Check sheet for the modelled part. Datum: model origin and axes. Units: mm. A direction names the side the tool comes from. Give positions to 0.01 mm unless a question says otherwise; leave off trailing zeros. Loops run counter-clockwise (first coordinate to the right, second up) from the corner with the lowest first, then second, coordinate; pieces in that order, holes last. Notation, with made-up numbers: (86, 78) -> (138, 78) arc R38 cw to (138, 116) -> close; hole circle Ø11 at (71, 64.25). An arc over 180 degrees is marked (long way). Answer as CSV lines item,"result". Start each with the question number.
(1) Section check B-B on z = 12. Enter the section's corners in (x, y), plus the area to 3 significant figures.
(2) Section check C-C on y = -13.5. Enter the section's corners in (x, z), plus the area to 3 significant figures.
(3) Section check D-D on z = 156.5. Enter the section's corners in (x, y) (1 decimal).
(4) Access from +Z, -Z, +X, -X, +Y, -Y to the whole of each face (thin tool, end or side, straight path). Record for faces 3 (the face through (2, -2, 0)), 4 (the face through (-2, 0, 2.4)).
(5) Material ranges on line 1 (Y direction, x = 0, z = 0.6); line 2 (Z direction, x = 2.75, y = -7); line 3 (X direction, y = -113, z = 156.5), recorded low to high. Write a range as from..to.
(6) Gauge pin test, flat ends, axial feed: pin 1 Ø2 at (y, z) = (-72.5, 121) entering from -X; pin 2 Ø6 at (x, y) = (13.5, -64) entering from -Z; pin 3 Ø2 at (y, z) = (-0.5, 6.5) entering from +X. Record the tip position at first contact, or that the pin passes through.
(7) Release check for a two-part mould opening along Y. For faces 1 (the face through (0, -118, 135)), 2 (the face through (0.54, -2.44, 1.18)) record: pulls with the +Y half, pulls with the -Y half, needs draft (parallel to the pull), parting line crosses it, or undercut.
(8) Section check A-A on x = 12. Enter the section's corners in (y, z).
Autodesk Inventor part; units mm, degrees
ref_plane "YZ Plane" through (0, 0, 0) normal (1, 0, 0) x (0, 1, 0)
ref_plane "XZ Plane" through (0, 0, 0) normal (0, 1, 0) x (-1, 0, 0)
ref_plane "XY Plane" through (0, 0, 0) normal (0, 0, 1) x (1, 0, 0)
sketch "Эскиз1" plane through (0, 0, 0) normal (0, 0, 1) x (1, 0, 0)
  circle A0 centre (0, 0) radius 4.6
  dimension "d0" = 9.2
extrude "Выдавливание1" add sketch "Эскиз1" along normal blind 170
sketch "Эскиз3" plane through (0, 0, 170) normal (0, 0, 1) x (1, 0, 0)
  circle A0 centre (0, 0) radius 4.6
  arc A1 (0, -114.6) -> (0, -4.6) centre (-83.8186, -59.6) ccw
  arc A2 (0, -121.5921) -> (3.6237, -2.8336) centre (-83.8186, -59.6) ccw
  line L0 (0, 0) -> (0, -4.6) construction
  line L1 (0, -114.6) -> (0, -121.5921)
  dimension "d3" = 4
  dimension "d4" = 110
extrude "Выдавливание2" add sketch "Эскиз3" against normal blind 70 contours A0 A2 L1 A1
sketch "Эскиз5" plane through (0, 0, 0) normal (0, 0, -1) x (-1, 0, 0)
  line L0 (-1.5, 1.3229) -> (-1.5, -1.3229)
  arc A0 (1.5, 1.3229) -> (-1.5, 1.3229) centre (0, 0) ccw
  line L1 (1.5, -1.3229) -> (1.5, 1.3229)
  arc A1 (-1.5, -1.3229) -> (1.5, -1.3229) centre (0, 0) ccw
  point P0 (0, 0)
extrude "Выдавливание4" cut sketch "Эскиз5" against normal blind 8.4
sketch "Эскиз6" plane through (0, 0, 0) normal (0, 0, -1) x (-1, 0, 0)
  circle A0 centre (0, 0) radius 2.5
  point P0 (0, 0)
extrude "Выдавливание5" cut sketch "Эскиз6" against normal blind 2.4
properties part number "локатор"
Working result:
1,outline,"circle Ø9.2 at (0, 0)"
1,area,"66.5 mm^2"
2,outline,"(5.21, 100) -> (9.69, 100) -> (9.69, 170) -> (5.21, 170) -> close"
2,area,"314 mm^2"
3,outline,"(0, -121.6) arc R104.3 ccw to (3.6, -2.8) arc R4.6 ccw (long way) to (0, -4.6) arc R100.3 cw to (0, -114.6) -> close"
4,face 3,"-Z, +X, -X, +Y, -Y"
4,face 4,"-Z"
5,line 1,"y = -4.6..-2.5, 2.5..4.6"
5,line 2,"z = 100..170"
5,line 3,"x = 1.03..5.72"
6,pin 1,"stops at x = 15.47"
6,pin 2,"stops at z = 100"
6,pin 3,"stops at x = 4.6"
7,face 1,"needs draft"
7,face 2,"undercut"
8,outline,"(-100.68, 100) -> (-89.08, 100) -> (-89.08, 170) -> (-100.68, 170) -> close; (-30.12, 100) -> (-18.52, 100) -> (-18.52, 170) -> (-30.12, 170) -> close"
